Model file for the job. Use its own axes, mm. Round coordinates to 2 decimals unless told otherwise and drop trailing zeros. Write each loop counter-clockwise with the first axis right and the second up, starting at its lowest first coordinate (ties: lowest second). Pieces come first, ordered by that corner, then holes. Notation, with made-up numbers: (45.5, -36.5) - (59.5, -36.5) arc R27 ccw to (59.5, 0.5) - close; hole circle Ø6 at (48.25, 72). An arc over 180 degrees is marked (long way). Answer as a JSON object with one key per item and string values. Group by question number.
from build123d import *

# Parameters (mm, degrees)
SKETCH2_R            = 60
SKETCH2_R_2          = 45
BOSS_EXTRUDE2_DEPTH  = 25
SKETCH3_R            = 60
BOSS_EXTRUDE3_DEPTH  = 5
M6_CLEARANCE_HOLE1_D = 6.6


with BuildPart() as part:
    # Sketch2 → Boss-Extrude2 (new body, symmetric)
    with BuildSketch(Plane.XY):
        Circle(SKETCH2_R)
        Circle(SKETCH2_R_2, mode=Mode.SUBTRACT)
    extrude(amount=BOSS_EXTRUDE2_DEPTH, both=True)

    # Sketch3 → Boss-Extrude3 (add)
    with BuildSketch(Plane.XY.offset(25)):
        Circle(SKETCH3_R)
        with BuildLine():
            ThreePointArc((24.990710007, 16.9559551), (22.605024595, 20.026304279), (19.844624318, 22.764685055))
            ThreePointArc((19.844624318, 22.764685055), (18.973362541, 27.487661121), (14.248349522, 26.62751464))
            ThreePointArc((14.248349522, 26.62751464), (10.709067589, 28.237490529), (6.99226553, 29.379384316))
            ThreePointArc((6.99226553, 29.379384316), (4.025925121, 33.156476395), (0.241863872, 30.199031472))
            ThreePointArc((0.241863872, 30.199031472), (-3.640207744, 29.979807998), (-7.461937025, 29.263620689))
            ThreePointArc((-7.461937025, 29.263620689), (-11.843803227, 31.229542506), (-13.820029875, 26.852314132))
            ThreePointArc((-13.820029875, 26.852314132), (-17.155555351, 24.85411275), (-20.206699734, 22.443914227))
            ThreePointArc((-20.206699734, 22.443914227), (-25.000258989, 22.148296785), (-24.715921328, 17.35405523))
            ThreePointArc((-24.715921328, 17.35405523), (-26.740771975, 14.034639796), (-28.322351051, 10.482577495))
            ThreePointArc((-28.322351051, 10.482577495), (-32.429456702, 7.993143187), (-29.949693064, 3.880191413))
            ThreePointArc((-29.949693064, 3.880191413), (-30.2, 0), (-29.949693064, -3.880191413))
            ThreePointArc((-29.949693064, -3.880191413), (-32.429456702, -7.993143187), (-28.322351051, -10.482577495))
            ThreePointArc((-28.322351051, -10.482577495), (-26.740771975, -14.034639796), (-24.715921328, -17.35405523))
            ThreePointArc((-24.715921328, -17.35405523), (-25.000258989, -22.148296785), (-20.206699734, -22.443914227))
            ThreePointArc((-20.206699734, -22.443914227), (-17.155555351, -24.85411275), (-13.820029875, -26.852314132))
            ThreePointArc((-13.820029875, -26.852314132), (-11.843803227, -31.229542506), (-7.461937025, -29.263620689))
            ThreePointArc((-7.461937025, -29.263620689), (-3.640207744, -29.979807998), (0.241863872, -30.199031472))
            ThreePointArc((0.241863872, -30.199031472), (4.025925121, -33.156476395), (6.99226553, -29.379384316))
            ThreePointArc((6.99226553, -29.379384316), (10.709067589, -28.237490529), (14.248349522, -26.62751464))
            ThreePointArc((14.248349522, -26.62751464), (18.973362541, -27.487661121), (19.844624318, -22.764685055))
            ThreePointArc((19.844624318, -22.764685055), (22.605024595, -20.026304279), (24.990710007, -16.9559551))
            ThreePointArc((24.990710007, -16.9559551), (29.574231257, -15.521753946), (28.150818829, -10.934870793))
            ThreePointArc((28.150818829, -10.934870793), (29.322442886, -7.227333061), (30.008, -3.399990588))
            ThreePointArc((30.008, -3.399990588), (33.4, 0), (30.008, 3.399990588))
            ThreePointArc((30.008, 3.399990588), (29.322442886, 7.227333061), (28.150818829, 10.934870793))
            ThreePointArc((28.150818829, 10.934870793), (29.574231257, 15.521753946), (24.990710007, 16.9559551))
        make_face(mode=Mode.SUBTRACT)
    extrude(amount=BOSS_EXTRUDE3_DEPTH)

    # M6 Clearance Hole1 (through all)
    with Locations(Plane.XY.offset(30)):
        with Locations((-37.123106012, 37.123106012), (0, 52.5), (37.123106012, 37.123106012), (52.5, 0), (37.123106012, -37.123106012), (0, -52.5), (-37.123106012, -37.123106012), (-52.5, 0)):
            Hole(M6_CLEARANCE_HOLE1_D / 2)


solid = part.part
(1) Slice it at D-D (z = -18). Count the separate pieces of the cut face and the enclosed holes in it, then the cut area to 3 significant figures.
(2) Pull direction Y, two halves, no side cores. Call faces 1 (the cylindrical face through (19.034, 27.445, 27.465)), 2 (the flat face through (22, -40, -25)): pulls with the +Y half, pulls with the -Y half, needs draft (parallel to the pull), parting line crosses it, or undercut.
(3) Flat gauge pins, fed straight in: pin 1 (5 mm diameter, centred on y = 24.5, z = -7.5, fed in from +X); pin 2 (4 mm diameter, centred on x = -6, y = -41, fed in from -Z); pin 3 (8 mm diameter, centred on y = -14.5, z = -2.5, fed in from +X). Where does each tip first touch, or does it go through?
(4) Slice it at A-A (y = 0). Write the cut outline in (x, z), then the cut area to 3 significant figures.
(5) Drill centre lines: line 1 (Y direction, x = 0, z = 5); line 2 (X direction, y = 35, z = 28); line 3 (Y direction, x = -2, z = 7). Where is each one in solid material? Low to high. Write a range as from..to.
(6) Slice it at B-B (x = 52.5). Write the cut outline in (y, z).
Answer:
{
 "1": {"separate pieces": "1", "enclosed holes": "9", "area": "4,670 mm²"},
 "2": {"face 1": "undercut", "face 2": "needs draft"},
 "3": {"pin 1": "x = 55.82", "pin 2": "z = 25", "pin 3": "x = 59.07"},
 "4": {"outline": "(-60, -25) - (-55.8, -25) - (-55.8, 30) - (-60, 30) - close; (-49.2, -25) - (-45, -25) - (-45, 25) - (-30.2, 25) - (-30.2, 30) - (-49.2, 30) - close; (33.4, 25) - (45, 25) - (45, -25) - (49.2, -25) - (49.2, 30) - (33.4, 30) - close; (55.8, -25) - (60, -25) - (60, 30) - (55.8, 30) - close", "area": "1,060 mm²"},
 "5": {"line 1": "-60..-55.8, -49.2..-45, 45..49.2, 55.8..60", "line 2": "-48.73..-39.65, -34.6..34.6, 39.65..48.73", "line 3": "-59.97..-55.12, -49.88..-44.96, 44.96..49.88, 55.12..59.97"},
 "6": {"outline": "(-29.05, -25) - (-3.3, -25) - (-3.3, 30) - (-29.05, 30) - close; (3.3, -25) - (29.05, -25) - (29.05, 30) - (3.3, 30) - close"}
}
